from build123d import *

# Parameters (mm, degrees)
SKETCH1_W           = 117.348
SKETCH1_H           = 112.522
BOSS_EXTRUDE1_DEPTH = 2.794
SKETCH3_W           = 114.554
SKETCH3_H           = 2.794
BOSS_EXTRUDE2_DEPTH = 48.26
LPATTERN1_COUNT     = 2
LPATTERN1_PITCH     = 109.728
SKETCH4_W           = 2.794
SKETCH4_H           = 106.934
BOSS_EXTRUDE3_DEPTH = 48.26
SKETCH6_W           = 2.794
SKETCH6_H           = 112.522
BOSS_EXTRUDE4_DEPTH = 48.26


with BuildPart() as part:
    # Sketch1 → Boss-Extrude1 (new body)
    with BuildSketch(Plane(origin=(0, 0, 0), x_dir=(1, 0, 0), z_dir=(0, 1, 0))):
        with Locations((58.674, 56.261)):
            Rectangle(SKETCH1_W, SKETCH1_H)
    extrude(amount=BOSS_EXTRUDE1_DEPTH)

    # Sketch3 → Boss-Extrude2 (add)
    with BuildSketch(Plane(origin=(0, 2.794, 0), x_dir=(1, 0, 0), z_dir=(0, 1, 0))):
        with Locations((57.277, 1.397)):
            Rectangle(SKETCH3_W, SKETCH3_H)
    boss_extrude2 = extrude(amount=BOSS_EXTRUDE2_DEPTH)

    # LPattern1: Boss-Extrude2 ×2
    with Locations(*[(0, 0, -i * LPATTERN1_PITCH) for i in range(1, LPATTERN1_COUNT)]):
        add(boss_extrude2)

    # Sketch4 → Boss-Extrude3 (add)
    with BuildSketch(Plane(origin=(0, 2.794, 0), x_dir=(1, 0, 0), z_dir=(0, 1, 0))):
        with Locations((1.397, 56.261)):
            Rectangle(SKETCH4_W, SKETCH4_H)
    extrude(amount=BOSS_EXTRUDE3_DEPTH)

    # Sketch6 → Boss-Extrude4 (add)
    with BuildSketch(Plane(origin=(0, 2.794, 0), x_dir=(1, 0, 0), z_dir=(0, 1, 0))):
        with Locations((115.951, 56.261)):
            Rectangle(SKETCH6_W, SKETCH6_H)
    extrude(amount=BOSS_EXTRUDE4_DEPTH)


solid = part.part
Geometry check sheet. Reference: the model listing, model coordinates, mm. A direction names the side the tool comes from. Coordinates: 2 decimals unless noted, no trailing zeros. Order: outer loops, then holes, each group sorted by start corner. A loop starts at its lowest first (then second) coordinate and runs counter-clockwise, first axis right, second up. Notation, with made-up numbers: (-33.5, 83.5) - (0.5, 83.5) arc R28 cw to (0.5, 121.5) - close; hole circle Ø10 at (55.25, 28). An arc over 180 degrees is marked (long way). Answer in a Markdown table with one row per item. Add a question column.
1) Set-up check for faces 1 (the flat face through (114.554, 27, -56)), 2 (the flat face through (58, 0, -57)): record each of +Z, -Z, +X, -X, +Y, -Y from which the full face is reachable in a straight line by a thin tool's end or side.
2) Gauge pin test, flat end, axial feed: P1, Ø8, axis at x = 32, z = -35.5, coming from the +Y side. Record the tip position at first contact, or that the pin passes through.
3) Cross-section at A-A, the plane x = 40. Record the cut outline in (y, z).
4) Release check for a two-part mould opening along Z. For faces 3 (the flat face through (58, 25, 0)), 4 (the flat face through (58, 25, -112.522)), 5 (the flat face through (58, 27, -2.794)) record: +Z half, -Z half, draft (parallel to the pull), parting line (faces both ways), or undercut.
5) Material ranges on line 1 along Z through (x, y) = (50.5, 27.5); line 2 along X through (y, z) = (15, -106); line 3 along Y through (x, z) = (36, -26), recorded low to high. Write a range as [from, to].
6) Cross-section at C-C, the plane z = -96. Record the cut outline in (x, y), then the cut area to 3 significant figures.
7) Cross-section at B-B, the plane y = 48.5. Record the cut outline in (x, z).
Check result:
| question | item | result |
|---|---|---|
| 1 | face 1 | +Y |
| 1 | face 2 | +Z, -Z, +X, -X, -Y |
| 2 | P1 | stops at y = 2.79 |
| 3 | outline | (0, -112.52) - (51.05, -112.52) - (51.05, -109.73) - (2.79, -109.73) - (2.79, -2.79) - (51.05, -2.79) - (51.05, 0) - (0, 0) - close |
| 4 | face 3 | +Z half |
| 4 | face 4 | -Z half |
| 4 | face 5 | undercut |
| 5 | line 1 | z = [-112.52, -109.73], [-2.79, 0] |
| 5 | line 2 | x = [0, 2.79], [114.55, 117.35] |
| 5 | line 3 | y = [0, 2.79] |
| 6 | outline | (0, 0) - (117.35, 0) - (117.35, 51.05) - (114.55, 51.05) - (114.55, 2.79) - (2.79, 2.79) - (2.79, 51.05) - (0, 51.05) - close |
| 6 | area | 598 mm² |
| 7 | outline | (0, -112.52) - (117.35, -112.52) - (117.35, 0) - (0, 0) - close; hole (2.79, -109.73) - (114.55, -109.73) - (114.55, -2.79) - (2.79, -2.79) - close |
